```python
from build123d import *

# Parameters (mm, degrees)
SKETCH1_W            = 60
SKETCH1_H            = 25
BASE_DEPTH           = 10
PEN_HOLE_REACH       = 24
SKETCH5_R            = 6.15
STAB_FINS_DEPTH      = 4
STAB_FINS_DEPTH_BACK = 4
BASE_DEC_R           = 4
SKETCH8_R            = 2
CUT_EXTRUDE2_DEPTH   = 23
CHAMFER1_SIZE        = 2


with BuildPart() as part:
    # Sketch1 → Base (new body)
    with BuildSketch(Plane(origin=(0, 0, 0), x_dir=(1, 0, 0), z_dir=(0, 1, 0))):
        Rectangle(SKETCH1_W, SKETCH1_H)
    extrude(amount=BASE_DEPTH)

    # Sketch2 → Pen Catch (revolve)
    with BuildSketch(Plane.XY):
        Polygon((-6.15, 0), (-6.15, -7), (-5.4, -7), (-5.4, -12), (-12, -12), (-12, 0), align=None)
    revolve(axis=Axis((0, 0, 0), (0, -1, 0)))

    # Sketch5 → Pen Hole (cut, up to next)
    with BuildSketch(Plane(origin=(0, 10, 0), x_dir=(1, 0, 0), z_dir=(0, 1, 0)), mode=Mode.PRIVATE) as pen_hole_sk1:
        Circle(SKETCH5_R)
    pen_hole_tool1 = extrude(pen_hole_sk1.sketch, amount=-PEN_HOLE_REACH, mode=Mode.PRIVATE) & part.part
    add(pen_hole_tool1.solids().sort_by_distance((0, 10, 0))[0], mode=Mode.SUBTRACT)

    # Sketch4 → Stab Fins (add, two sides)
    with BuildSketch(Plane.XY) as stab_fins_sk:
        Polygon((-22, 0), (-10, 0), (-10, -12), align=None)
        Polygon((10, -12), (22, 0), (10, 0), align=None)
    extrude(amount=STAB_FINS_DEPTH)
    extrude(stab_fins_sk.sketch, amount=-STAB_FINS_DEPTH_BACK)

    # Base Dec
    base_dec_edges = [part.edges().sort_by_distance(p)[0] for p in [
        (-30, 5, -12.5),
        (30, 5, -12.5),
        (30, 5, 12.5),
        (-30, 5, 12.5),
    ]]
    fillet(base_dec_edges, radius=BASE_DEC_R)

    # Sketch8 → Cut-Extrude2 (cut, through all)
    with BuildSketch(Plane(origin=(0, 10, 0), x_dir=(1, 0, 0), z_dir=(0, 1, 0))):
        with Locations((23.15, 9.4)):
            Circle(SKETCH8_R)
        with Locations((23.15, -9.4)):
            Circle(SKETCH8_R)
        with Locations((-23.15, 9.4)):
            Circle(SKETCH8_R)
        with Locations((-23.15, -9.4)):
            Circle(SKETCH8_R)
    extrude(amount=-CUT_EXTRUDE2_DEPTH, mode=Mode.SUBTRACT)

    # Chamfer1
    chamfer1_edges = [part.edges().sort_by_distance(p)[0] for p in [
        (5.4, -12, 0),
    ]]
    chamfer(chamfer1_edges, length=CHAMFER1_SIZE)


solid = part.part
```
CAD build for the part. Positions are in the model's coordinates, mm. A direction names the side the tool comes from. Give positions to 0.01 mm unless a question says otherwise; leave off trailing zeros. Loops run counter-clockwise (first coordinate to the right, second up) from the corner with the lowest first, then second, coordinate; pieces in that order, holes last. Notation, with made-up numbers: (-22, 53) - (30, 53) arc R27 ccw to (30, 80) - close; hole circle Ø11 at (55.5, 45). An arc over 180 degrees is marked (long way). Put each result on its own line as item: value.
Q1. Mould opens along X. For faces 1 (the face through (25.058, 5.07, 8.799)), 2 (the face through (15, -4, -4)), 3 (the face through (-28.797, 5.07, -11.359)) say: pulls with the +X half, pulls with the -X half, needs draft (parallel to the pull), parting line crosses it, or undercut.
Filled in:
face 1: undercut
face 2: needs draft
face 3: pulls with the -X half
Q2. Slice it at C-C (y = -7.75). Give the cut face in (x, z).
Filled in:
outline: (-14.25, -4) - (-11.31, -4) arc R12 ccw to (11.31, -4) - (14.25, -4) - (14.25, 4) - (11.31, 4) arc R12 ccw to (-11.31, 4) - (-14.25, 4) - close; hole circle Ø10.8 at (0, 0)
Q3. Slice it at A-A (x = -23.15). Give the cut face in (y, z), plus the area to 3 significant figures.
Filled in:
outline: (0, -12.5) - (10, -12.5) - (10, -11.4) - (0, -11.4) - close; (0, -7.4) - (10, -7.4) - (10, 7.4) - (0, 7.4) - close; (0, 11.4) - (10, 11.4) - (10, 12.5) - (0, 12.5) - close
area: 170 mm²
Q4. Slice it at B-B (z = 0). Give the cut face in (x, y).
Filled in:
outline: (-30, 0) - (-22, 0) - (-12, -10) - (-12, -12) - (-7.4, -12) - (-5.4, -10) - (-5.4, -7) - (-6.15, -7) - (-6.15, 10) - (-30, 10) - close; (5.4, -10) - (7.4, -12) - (12, -12) - (12, -10) - (22, 0) - (30, 0) - (30, 10) - (6.15, 10) - (6.15, -7) - (5.4, -7) - close
Q5. Flat gauge pins, fed straight in: pin 1 (3.5 mm diameter, centred on x = 1.5, z = 1, fed in from +Y); pin 2 (3 mm diameter, centred on x = 19, y = -4.5, fed in from +Z); pin 3 (12 mm diameter, centred on x = -15.5, y = -7, fed in from -Z); pin 4 (1.5 mm diameter, centred on x = -22, z = 6, fed in from -Y). Where does each tip first touch, or does it go through?
Filled in:
pin 1: passes through
pin 2: stops at z = 4
pin 3: stops at z = -7.33
pin 4: stops at y = 0
Q6. Slice it at D-D (x = 0). Give the cut face in (y, z).
Filled in:
outline: (-12, -12) - (0, -12) - (0, -12.5) - (10, -12.5) - (10, -6.15) - (-7, -6.15) - (-7, -5.4) - (-10, -5.4) - (-12, -7.4) - close; (-12, 7.4) - (-10, 5.4) - (-7, 5.4) - (-7, 6.15) - (10, 6.15) - (10, 12.5) - (0, 12.5) - (0, 12) - (-12, 12) - close
Q7. Probe line 1 along Z through (x, y) = (-23.15, 7.5); line 2 along Z through (x, y) = (0, 0.5); line 3 along X through (y, z) = (4.25, 9.4). List the from-to ranges inside material, lowest first.
Filled in:
line 1: z = -12.5 to -11.4, -7.4 to 7.4, 11.4 to 12.5
line 2: z = -12.5 to -6.15, 6.15 to 12.5
line 3: x = -29.9 to -25.15, -21.15 to 21.15, 25.15 to 29.9
Q8. Tool access for faces 4 (the face through (-5.537, -5.916, 10.646)), 5 (the face through (15, -4, 4)), 6 (the face through (-15, -4, -4)), 7 (the face through (0.405, 1.619, -6.137)): list every direction of +Z, -Z, +X, -X, +Y, -Y with a clear straight run to the whole face (end or side of a thin tool).
Filled in:
face 4: -Y
face 5: +Z, +X, -Y
face 6: -Z, -X, -Y
face 7: +Y
